Check sheet for the modelled part. Datum: model origin and axes. Units: mm. A direction names the side the tool comes from. Round coordinates to 2 decimals unless told otherwise and drop trailing zeros. Write each loop counter-clockwise with the first axis right and the second up, starting at its lowest first coordinate (ties: lowest second). Pieces come first, ordered by that corner, then holes.
Item 1: Cross-section at C-C on x = 53. Enter the section's corners in (y, z).
Item 2: Cross-section at A-A on z = 69.85. Enter the section's corners in (x, y), plus the area to 3 significant figures.
Item 3: Cross-section at B-B on x = 38.1. Count the separate pieces of the cut face and the enclosed holes in it, plus the area to 3 significant figures.
Item 4: Go/stop test with flat-tipped pins: pin 1 Ø1.9 at (x, z) = (45.5, 21.5) entering from +Y; pin 2 Ø5.5 at (x, z) = (38.1, 69.85) entering from -Y. Record where each tip stops, or that it passes through.
Item 5: Tool access check on faces 1 (the cylindrical face through (38.54, 2.03, 66.5)), 2 (the flat face through (38, 3.492, 43)). Record the directions out of +Z, -Z, +X, -X, +Y, -Y that give a thin tool (end or side, any length) a straight path to the whole face; none if there is none.
Item 6: Cross-section at D-D on z = 90.5. Enter the section's corners in (x, y).
Item 7: Release check for a two-part mould opening along Z. For faces 3 (the cylindrical face through (74.39, 2.41, 1.91)), 4 (the flat face through (38, 3.492, 92)), 5 (the flat face through (76.2, 2, 51)) record: +Z half, -Z half, draft (parallel to the pull), parting line (faces both ways), or undercut.
Item 8: Material ranges on line 1 (Z direction, x = 38.1, y = 1.7); line 2 (X direction, y = 1.95, z = 31.75); line 3 (Y direction, x = 65, z = 62), recorded low to high.
from build123d import *

# Parameters (mm, degrees)
SKETCH1_W                         = 76.2
SKETCH1_H                         = 101.6
BOSS_EXTRUDE1_DEPTH               = 4.7625
F_1_4_CLEARANCE_HOLE1_D           = 6.7564
F_1_4_CLEARANCE_HOLE1_CSINK_D     = 8.0264
F_1_4_CLEARANCE_HOLE1_CSINK_ANGLE = 90
FILLET1_R                         = 6.35
SKETCH7_W                         = 76.2
SKETCH7_H                         = 6.35
CUT_EXTRUDE1_DEPTH                = 1.27


with BuildPart() as part:
    # Sketch1 → Boss-Extrude1 (new body)
    with BuildSketch(Plane(origin=(0, 0, 0), x_dir=(1, 0, 0), z_dir=(0, 1, 0))):
        with Locations((38.1, -50.8)):
            Rectangle(SKETCH1_W, SKETCH1_H)
    extrude(amount=BOSS_EXTRUDE1_DEPTH)

    # 1/4 Clearance Hole1 (through all)
    with Locations(Plane(origin=(0, 4.7625, 0), x_dir=(1, 0, 0), z_dir=(0, 1, 0))):
        with Locations((38.1, -69.85), (38.1, -31.75)):
            CounterSinkHole(F_1_4_CLEARANCE_HOLE1_D / 2, F_1_4_CLEARANCE_HOLE1_CSINK_D / 2, counter_sink_angle=F_1_4_CLEARANCE_HOLE1_CSINK_ANGLE)

    # Fillet1
    fillet1_edges = [part.edges().sort_by_distance(p)[0] for p in [
        (0, 2.38125, 0),
        (76.2, 2.38125, 0),
        (76.2, 2.38125, 101.6),
        (0, 2.38125, 101.6),
    ]]
    fillet(fillet1_edges, radius=FILLET1_R)

    # Sketch7 → Cut-Extrude1 (cut)
    with BuildSketch(Plane(origin=(0, 4.7625, 0), x_dir=(1, 0, 0), z_dir=(0, 1, 0))):
        with Locations((38.1, -9.525)):
            Rectangle(SKETCH7_W, SKETCH7_H)
        with Locations((38.1, -42.545)):
            Rectangle(SKETCH7_W, SKETCH7_H)
        with Locations((38.1, -59.055)):
            Rectangle(SKETCH7_W, SKETCH7_H)
        with Locations((38.1, -92.075)):
            Rectangle(SKETCH7_W, SKETCH7_H)
        with Locations((38.1, -79.375)):
            Rectangle(SKETCH7_W, SKETCH7_H)
        with Locations((38.1, -22.225)):
            Rectangle(SKETCH7_W, SKETCH7_H)
    extrude(amount=-CUT_EXTRUDE1_DEPTH, mode=Mode.SUBTRACT)


solid = part.part
Response values:
1. outline: (0, 0) - (4.76, 0) - (4.76, 6.35) - (3.49, 6.35) - (3.49, 12.7) - (4.76, 12.7) - (4.76, 19.05) - (3.49, 19.05) - (3.49, 25.4) - (4.76, 25.4) - (4.76, 39.37) - (3.49, 39.37) - (3.49, 45.72) - (4.76, 45.72) - (4.76, 55.88) - (3.49, 55.88) - (3.49, 62.23) - (4.76, 62.23) - (4.76, 76.2) - (3.49, 76.2) - (3.49, 82.55) - (4.76, 82.55) - (4.76, 88.9) - (3.49, 88.9) - (3.49, 95.25) - (4.76, 95.25) - (4.76, 101.6) - (0, 101.6) - close
2. outline: (0, 0) - (34.72, 0) - (34.72, 4.13) - (34.09, 4.76) - (0, 4.76) - close; (41.48, 0) - (76.2, 0) - (76.2, 4.76) - (42.11, 4.76) - (41.48, 4.13) - close
2. area: 330 mm2
3. separate pieces: 3
3. enclosed holes: 0
3. area: 370 mm2
4. pin 1: stops at y = 3.49
4. pin 2: passes through
5. face 1: +Y, -Y
5. face 2: +X, -X, +Y
6. outline: (0, 0) - (76.2, 0) - (76.2, 3.49) - (0, 3.49) - close
7. face 3: -Z half
7. face 4: undercut
7. face 5: draft
8. line 1: z = 0 to 28.37, 35.13 to 66.47, 73.23 to 101.6
8. line 2: x = 0 to 34.72, 41.48 to 76.2
8. line 3: y = 0 to 3.49
